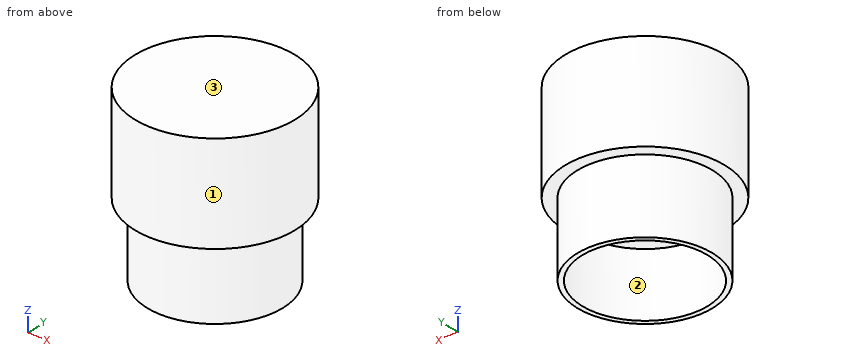
from build123d import *

# Parameters (mm, degrees)
SKETCH_R     = 13.75
PAD_DEPTH    = 15
SKETCH001_R  = 12.75
POCKET_DEPTH = 13
SKETCH002_R  = 16.25
PAD001_DEPTH = 20


with BuildPart() as part:
    # Sketch → Pad (new body)
    with BuildSketch(Plane.XY):
        Circle(SKETCH_R)
    extrude(amount=PAD_DEPTH)

    # Sketch001 (on Face2 of Pad) → Pocket (cut)
    with BuildSketch(Plane(origin=(0, 0, 0), x_dir=(1, 0, 0), z_dir=(0, 0, -1))):
        Circle(SKETCH001_R)
    extrude(amount=-POCKET_DEPTH, mode=Mode.SUBTRACT)

    # Sketch002 (on Face3 of Pocket) → Pad001 (join)
    with BuildSketch(Plane.XY.offset(15)):
        Circle(SKETCH002_R)
    extrude(amount=PAD001_DEPTH)


solid = part.part
Read the model definition and answer for the solid it produces. Units are mm, in the model's axes. Face numbers are marked on the shaded views. Round coordinates to 2 decimals unless told otherwise and drop trailing zeros. Order: outer loops, then holes, each group sorted by start corner. A loop starts at its lowest first (then second) coordinate and runs counter-clockwise, first axis right, second up.
1) The part is cut by section A-A on x = 0. Write down the section's boundary in (y, z), plus the area to 3 significant figures.
2) The part is cut by section D-D on z = 31. Write down the section's boundary in (x, y), plus the area to 3 significant figures.
3) Flat-ended cylindrical pins translate along their axes: pin 1 (1.5 mm diameter, centred on x = -10, z = 31, fed in from -Y); pin 2 (1 mm diameter, centred on y = -10.5, z = 13.5, fed in from +X); pin 3 (13 mm diameter, centred on x = 4.5, y = -3, fed in from -Z). Find the tip coordinate at first contact, or state that the pin passes through.
4) The mould has two halves that part along X. Classify the marked faces 1, 2 and 3: released by +X, released by -X, zero draft, split by the parting line, or undercut.
5) Straight lines are drawn through the part: L1, parallel to Y at x = 0, z = 9; L2, parallel to Z at x = 2.5, y = 5.5; L3, parallel to Z at x = 14, y = 3. For each, find the intervals that lie inside material, in ascending order.
6) The part is cut by section C-C on z = 9. Write down the section's boundary in (x, y).
Resolved:
1. outline: (-16.25, 15) - (-13.75, 15) - (-13.75, 0) - (-12.75, 0) - (-12.75, 13) - (12.75, 13) - (12.75, 0) - (13.75, 0) - (13.75, 15) - (16.25, 15) - (16.25, 35) - (-16.25, 35) - close
1. area: 731 mm2
2. outline: circle Ø32.5 at (0, 0)
2. area: 830 mm2
3. pin 1: stops at y = -13.36
3. pin 2: stops at x = 9.44
3. pin 3: stops at z = 13
4. face 1: split by the parting line
4. face 2: undercut
4. face 3: zero draft
5. L1: y = -13.75 to -12.75, 12.75 to 13.75
5. L2: z = 13 to 35
5. L3: z = 15 to 35
6. outline: circle Ø27.5 at (0, 0); hole circle Ø25.5 at (0, 0)
